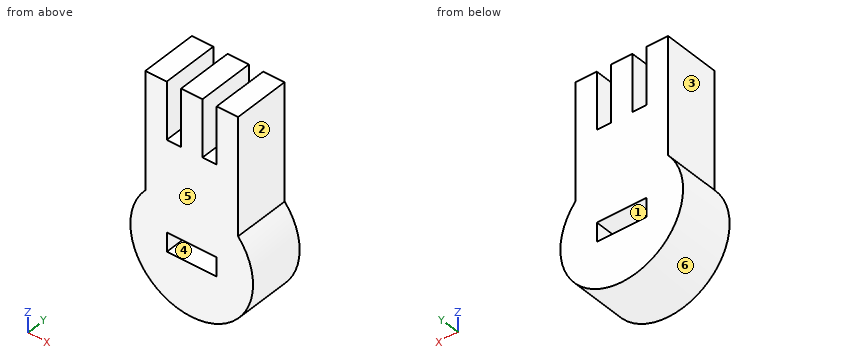
```python
from build123d import *

# Parameters (mm, degrees)
SKETCH1_W           = 3.5
SKETCH1_H           = 1.322228747
BOSS_EXTRUDE1_DEPTH = 4


with BuildPart() as part:
    # Sketch1 → Boss-Extrude1 (new body)
    with BuildSketch(Plane(origin=(0, 0, 0), x_dir=(1, 0, 0), z_dir=(0, 1, 0))):
        with BuildLine():
            Line((0, 0), (0, -4))
            Line((0, -4), (1.5, -4))
            Line((1.5, -4), (1.5, 0))
            Line((1.5, 0), (2.5, 0))
            Line((2.5, 0), (2.5, -4))
            Line((2.5, -4), (4, -4))
            Line((4, -4), (4, 0))
            Line((4, 0), (5, 0))
            Line((5, 0), (5, -4))
            Line((5, -4), (6.5, -4))
            Line((6.5, -4), (6.5, 0))
            Line((6.5, 0), (6.5, 4.184418355))
            ThreePointArc((6.5, 4.184418355), (3.25, 11.3), (0, 4.184418355))
            Line((0, 4.184418355), (0, 0))
        make_face()
        with Locations((3.25, 7.017797312)):
            Rectangle(SKETCH1_W, SKETCH1_H, mode=Mode.SUBTRACT)
    extrude(amount=BOSS_EXTRUDE1_DEPTH)


solid = part.part
```
Work out the finished part from the listing and answer in its coordinate system (mm). Face numbers are marked on the shaded views. A direction names the side the tool comes from. Round coordinates to 2 decimals unless told otherwise and drop trailing zeros. Order: outer loops, then holes, each group sorted by start corner. A loop starts at its lowest first (then second) coordinate and runs counter-clockwise, first axis right, second up.
Q1. A tool of negligible diameter and unlimited length cuts with its end or side. For the marked faces 1, 2 and 3, from which of +Z, -Z, +X, -X, +Y, -Y can it reach the whole face along a straight path? Write none if from no direction.
Solution:
face 1: +Y, -Y
face 2: +Z, +X, +Y, -Y
face 3: +Z, -X, +Y, -Y
Q2. The mould has two halves that part along X. Classify the marked faces 4, 5 and 6: pulls with the +X half, pulls with the -X half, needs draft (parallel to the pull), parting line crosses it, or undercut.
Solution:
face 4: undercut
face 5: needs draft
face 6: parting line crosses it
Q3. Find the intervals of material crossed by line 1 along X through (y, z) = (1.9, -7); line 2 along X through (y, z) = (1.5, -1.5); line 3 along Z through (x, y) = (2.25, 1.7), in increasing order.
Solution:
line 1: x = -1.05 to 1.5, 5 to 7.55
line 2: x = 0 to 6.5
line 3: z = -11.18 to -7.68, -6.36 to 0
Q4. Given pin 1 Ø4 at (x, z) = (0.5, -2) entering from -Y; pin 2 Ø0.8 at (x, y) = (2, 1.5) entering from +Z; pin 3 Ø1 at (y, z) = (3.5, -9) entering from +X; pin 4 Ø1.2 at (y, z) = (3, 1) entering from +X, each flat-ended and moving along its own axis, determine where each tip first touches the part or whether it passes through.
Solution:
pin 1: stops at y = 0
pin 2: stops at z = 0
pin 3: stops at x = 7.28
pin 4: stops at x = 6.5
Q5. A cutting plane is placed at B-B, the plane x = 3.25. Determine the outline of the cut face in (y, z), then the cut area to 3 significant figures.
Solution:
outline: (0, -11.3) - (4, -11.3) - (4, -7.68) - (0, -7.68) - close; (0, -6.36) - (4, -6.36) - (4, 4) - (0, 4) - close
area: 55.9 mm2
Q6. A cutting plane is placed at D-D, the plane z = -7. Determine the outline of the cut face in (x, y), then the cut area to 3 significant figures.
Solution:
outline: (-1.05, 0) - (1.5, 0) - (1.5, 4) - (-1.05, 4) - close; (5, 0) - (7.55, 0) - (7.55, 4) - (5, 4) - close
area: 20.4 mm2
Q7. A cutting plane is placed at C-C, the plane y = 2.15. Determine the outline of the cut face in (x, z).
Solution:
outline: (0, -4.18) arc R4.3 ccw (long way) to (6.5, -4.18) - (6.5, 4) - (5, 4) - (5, 0) - (4, 0) - (4, 4) - (2.5, 4) - (2.5, 0) - (1.5, 0) - (1.5, 4) - (0, 4) - close; hole (1.5, -7.68) - (5, -7.68) - (5, -6.36) - (1.5, -6.36) - close
Q8. A cutting plane is placed at A-A, the plane z = 3.25. Determine the outline of the cut face in (x, y), then the cut area to 3 significant figures.
Solution:
outline: (0, 0) - (1.5, 0) - (1.5, 4) - (0, 4) - close; (2.5, 0) - (4, 0) - (4, 4) - (2.5, 4) - close; (5, 0) - (6.5, 0) - (6.5, 4) - (5, 4) - close
area: 18.0 mm2
